Can you work these out from the model? Positions are in its coordinate system, mm. Coordinates: 2 decimals unless noted, no trailing zeros. Loops run counter-clockwise (first coordinate to the right, second up) from the corner with the lowest first, then second, coordinate; pieces in that order, holes last. Notation, with made-up numbers: (81.25, 21) -> (118.25, 21) arc R6 ccw to (118.25, 27) -> close; hole circle Ø6 at (65, 38.25). An arc over 180 degrees is marked (long way). Use one line per item in the form item = value. Start each with the question number.
(1) Imagine slicing it at A-A (z = -300). List the corners of the cut face in (x, y) for me, plus the area to 3 significant figures.
(2) I need wall thicknesses on line 1 (Z direction, x = 0, y = 4.3); line 2 (Z direction, x = -1, y = 1.15); line 3 (X direction, y = 1.5, z = -294). Which ranges of each line are inside material? Lowest first, please. Write a range as [from, to].
(3) Imagine slicing it at B-B (x = 0). List the corners of the cut face in (y, z) for me, plus the area to 3 significant figures.
(4) Imagine slicing it at C-C (y = 1.45). List the corners of the cut face in (x, z) for me, plus the area to 3 significant figures.
(5) I'm going to push a flat-ended pin straight in: pin 1 (2.5 mm diameter, centred on x = 0, z = -343.336, fed in from +Y). Where does the tip first touch, or does it pass through?
Autodesk Inventor part; units mm, degrees
ref_plane "XZ Plane" through (0, 0, 0) normal (0, 1, 0) x (-1, 0, 0)
ref_plane "XY Plane" through (0, 0, 0) normal (0, 0, 1) x (1, 0, 0)
sketch "Sketch1" plane through (0, 0, 0) normal (0, 1, 0) x (-1, 0, 0)
  line L0 (0, 0) -> (0, -343.336) construction
  line L1 (-4, 0) -> (-4, -343.336)
  line L2 (4, -343.336) -> (4, 0)
  arc A0 (4, 0) -> (-4, 0) centre (0, 0) ccw
  arc A1 (-4, -343.336) -> (4, -343.336) centre (0, -343.336) ccw
  circle A2 centre (0, 0) radius 1.5
  circle A3 centre (0, -343.336) radius 1.5
  line L3 (0, -315.436) -> (0, -248.336) construction
  line L4 (1.5, -315.436) -> (1.5, -248.336)
  line L5 (-1.5, -248.336) -> (-1.5, -315.436)
  arc A4 (-1.5, -315.436) -> (1.5, -315.436) centre (0, -315.436) ccw
  arc A5 (1.5, -248.336) -> (-1.5, -248.336) centre (0, -248.336) ccw
  line L6 (0, -343.336) -> (0, -423.336) construction
  line L7 (-4, -343.336) -> (-4, -423.336)
  line L8 (4, -423.336) -> (4, -343.336)
  arc A6 (4, -343.336) -> (-4, -343.336) centre (0, -343.336) ccw
  arc A7 (-4, -423.336) -> (4, -423.336) centre (0, -423.336) ccw
  point P0 (0, -171.668)
  point P1 (0, -281.886)
  point P2 (0, -383.336)
  dimension "d0" = 8
  dimension "d1" = 343.336
  dimension "d2" = 3
  dimension "d3" = 3
  dimension "d14" = 3
  dimension "d15" = 27.9
  dimension "d16" = 95
  dimension "d17" = 8
  dimension "d18" = 80
extrude "Extrusion1" add sketch "Sketch1" along normal blind 6
sketch "Sketch3" plane through (0, 6, 0) normal (0, 1, 0) x (1, 0, 0)
  line L0 (-4, 423.336) -> (-4, 0)
  line L1 (-4, 214.6062) -> (0, 206.0281)
  line L2 (0, 206.0281) -> (4, 214.6062)
  line L3 (4, 0) -> (4, 423.336)
  line L4 (-4, 423.336) -> (-4, 0)
  arc A0 (-4, 0) -> (4, 0) centre (0, 0) ccw
  line L5 (4, 0) -> (4, 423.336)
  arc A1 (4, 423.336) -> (-4, 423.336) centre (0, 423.336) ccw
  arc A2 (1.5, 315.436) -> (-1.5, 315.436) centre (0, 315.436) ccw
  line L6 (1.5, 315.436) -> (1.5, 248.336)
  arc A3 (-1.5, 248.336) -> (1.5, 248.336) centre (0, 248.336) ccw
  line L7 (-1.5, 248.336) -> (-1.5, 315.436)
  circle A4 centre (0, 343.336) radius 1.5
  circle A5 centre (0, 0) radius 1.5
  dimension "d21" = 25
  dimension "d22" = 25
extrude "Extrusion2" [suppressed]
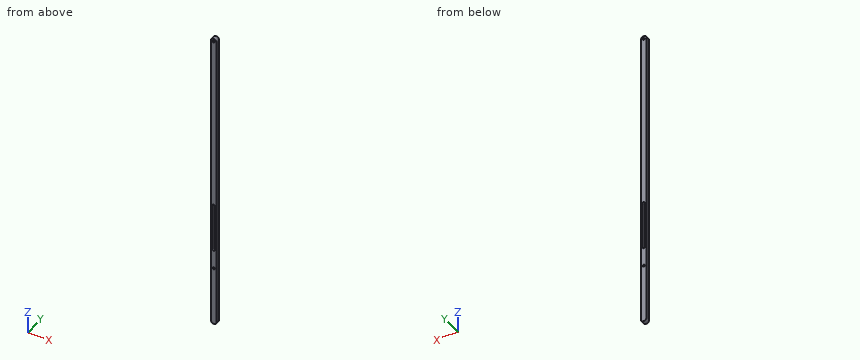
Worked out:
q1.outline = (-4, 0) -> (-1.5, 0) -> (-1.5, 6) -> (-4, 6) -> close; (1.5, 0) -> (4, 0) -> (4, 6) -> (1.5, 6) -> close
q1.area = 30.0 mm2
q2.line_1 = [-427.34, -344.84], [-341.84, -316.94], [-246.84, -1.5], [1.5, 4]
q2.line_2 = [-427.21, -344.45], [-342.22, -316.55], [-247.22, -1.12], [1.12, 3.87]
q2.line_3 = [-4, -1.5], [1.5, 4]
q3.outline = (0, -427.34) -> (6, -427.34) -> (6, -344.84) -> (0, -344.84) -> close; (0, -341.84) -> (6, -341.84) -> (6, -316.94) -> (0, -316.94) -> close; (0, -246.84) -> (6, -246.84) -> (6, -1.5) -> (0, -1.5) -> close; (0, 1.5) -> (6, 1.5) -> (6, 4) -> (0, 4) -> close
q3.area = 2,130 mm2
q4.outline = (-4, -423.34) arc R4 ccw to (4, -423.34) -> (4, 0) arc R4 ccw to (-4, 0) -> close; hole circle Ø3 at (0, -343.34); hole (-1.5, -315.44) arc R1.5 ccw to (1.5, -315.44) -> (1.5, -248.34) arc R1.5 ccw to (-1.5, -248.34) -> close; hole circle Ø3 at (0, 0)
q4.area = 3,210 mm2
q5.pin_1 = through
